Could you check a few things on this model? Use its own coordinates, in mm. A direction names the side the tool comes from. Coordinates: 2 decimals unless noted, no trailing zeros. Loops run counter-clockwise (first coordinate to the right, second up) from the corner with the lowest first, then second, coordinate; pieces in that order, holes last. Notation, with made-up numbers: M -31,40 L 3,40 A30 ccw 3,71 Z; hole C 60.5,15.5 d11. An arc over 180 degrees is marked long. Return JSON: item names as keys, results as strings. Group by question number.
Autodesk Inventor part; units mm, degrees
ref_plane "Work Plane1" through (120, 0, 0) normal (1, 0, 0) x (0, 1, 0)
ref_plane "Work Plane2" through (0, 0, 0) normal (0, 0, 1) x (1, 0, 0)
ref_plane "Work Plane3" through (0, 0, 0) normal (1, 0, 0) x (0, 1, 0)
sketch "Sketch1" plane through (0, 0, 0) normal (0, 0, 1) x (1, 0, 0)
  line L0 (0, 6) -> (0, 60)
  line L1 (0, 0) -> (0, 128.6868)
  arc A0 (0, 6) -> (6, 0) centre (6, 6) ccw
  line L2 (120, 0) -> (109.25, 0)
  line L3 (106.25, 3) -> (106.25, 5.75)
  line L4 (103.25, 8.75) -> (99.25, 8.75)
  line L5 (96.25, 5.75) -> (96.25, 3)
  line L6 (93.25, 0) -> (6, 0)
  arc A1 (93.25, 0) -> (96.25, 3) centre (93.25, 3) ccw
  arc A2 (99.25, 8.75) -> (96.25, 5.75) centre (99.25, 5.75) ccw
  arc A3 (106.25, 5.75) -> (103.25, 8.75) centre (103.25, 5.75) ccw
  arc A4 (106.25, 3) -> (109.25, 0) centre (109.25, 3) ccw
  point P0 (106.25, 0)
  point P1 (106.25, 8.75)
  point P2 (96.25, 8.75)
  dimension "d0" = 120
  dimension "d1" = 60
  dimension "d13" = 6
  dimension "d15" = 13.75
  dimension "d16" = 8.75
  dimension "d17" = 10
  dimension "d18" = 3
ref_plane "Work Plane1" through (120, 0, 0) normal (1, 0, 0) x (0, 1, 0)
sketch "Sketch2" plane through (120, 0, 0) normal (1, 0, 0) x (0, 1, 0)
  circle A0 centre (0, 0) radius 1.5
  point P0 (0, 0)
  dimension "d2" = 3
sweep "Sweep1" add profiles "Sketch2" path "Sketch1" path curves L2 A4 L3 A3 L4 A2 L5 A1 L6 A0 L0
thread "Thread1"
ref_plane "Work Plane2" through (0, 0, 0) normal (0, 0, 1) x (1, 0, 0)
thread "Thread2"
ref_plane "Work Plane3" through (0, 0, 0) normal (1, 0, 0) x (0, 1, 0)
properties part number "Barra en L"
(1) If I drill on L1, parallel to X at y = 27, z = -0.1; L2, parallel to X at y = 4.5, z = -0.15; L3, parallel to Y at x = 47.5, z = -0.2, over which ranges is the centre line in solid material (lowest first)? Write a range as [from, to].
(2) Imagine slicing it at B-B, the plane x = 32. Write out the boundary of the cut face in (y, z), then the cut area to 3 significant figures.
(3) For faces 1 (the face through (114.55, -1.5, -0.07)), 2 (the face through (94.82, 4.36, -0.45)), 3 (the face through (-1.5, 33.38, -0.07)), which set-ups out of +Z, -Z, +X, -X, +Y, -Y let a thin tool reach every point of the face, with its end or its side?
(4) Imagine slicing it at A-A, the plane z = 0. Write out the boundary of the cut face in (x, y).
Checks:
{
 "1": {"L1": "[-1.5, 1.5]", "L2": "[-1.34, 1.75], [94.76, 97.74], [104.76, 107.74]", "L3": "[-1.49, 1.49]"},
 "2": {"outline": "C 0,0 d3", "area": "7.07 mm²"},
 "3": {"face 1": "+X", "face 2": "none", "face 3": "+Y"},
 "4": {"outline": "M -1.5,6 A7.5 ccw 6,-1.5 L 93.25,-1.5 A4.5 ccw 97.75,3 L 97.75,5.75 A1.5 cw 99.25,7.25 L 103.25,7.25 A1.5 cw 104.75,5.75 L 104.75,3 A4.5 ccw 109.25,-1.5 L 120,-1.5 L 120,1.5 L 109.25,1.5 A1.5 cw 107.75,3 L 107.75,5.75 A4.5 ccw 103.25,10.25 L 99.25,10.25 A4.5 ccw 94.75,5.75 L 94.75,3 A1.5 cw 93.25,1.5 L 6,1.5 A4.5 cw 1.5,6 L 1.5,60 L -1.5,60 Z"}
}
